Answer from the drawing. Dimensions are ordinates in mm from the lowest x, y and z of the part. A direction names the side the tool comes from. Give positions to 0.01 mm unless a question says otherwise; leave off trailing zeros. Write each loop counter-clockwise with the first axis right and the second up, starting at its lowest first coordinate (ties: lowest second). Pieces come first, ordered by that corner, then holes.
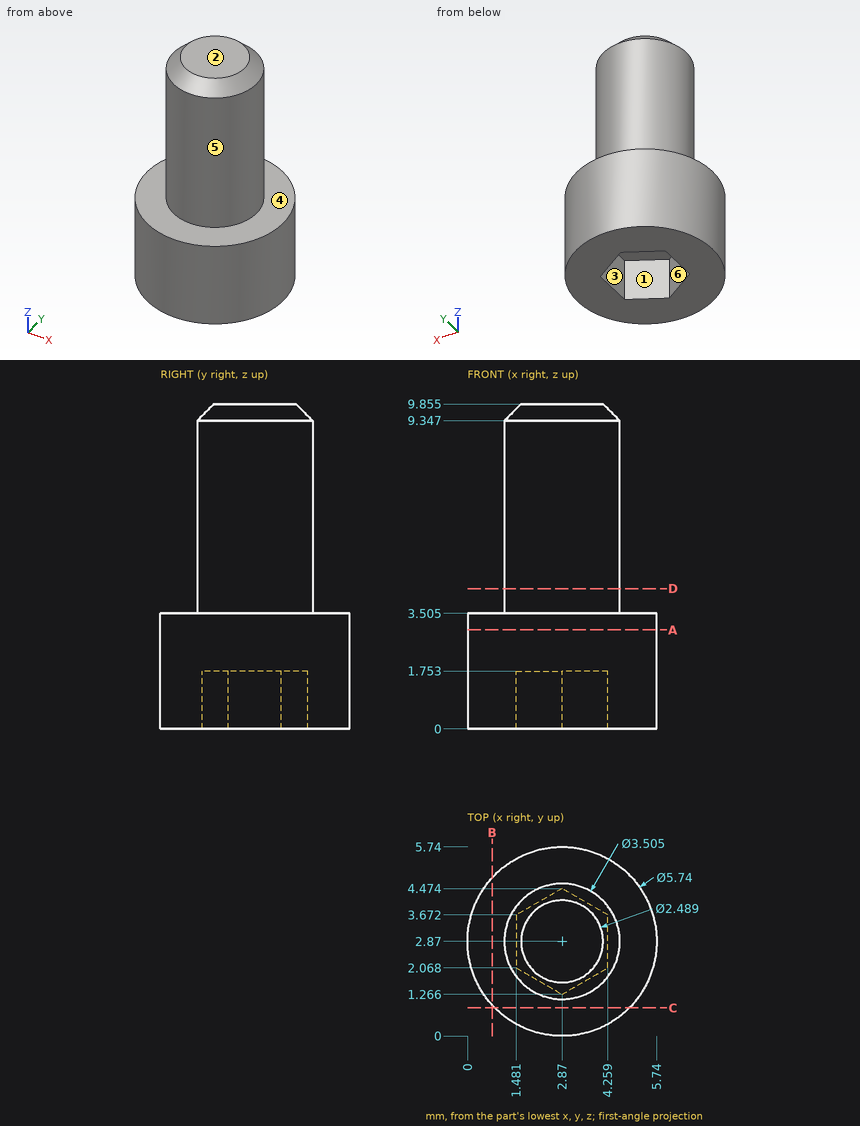
Item 1: A cutting plane is placed at C-C, the plane y = 0.85. Give the vertices of the cut face in (x, z) (1 decimal), plus the area to 3 significant figures.
Conclusion:
outline: (0.8, 0) - (4.9, 0) - (4.9, 3.5) - (0.8, 3.5) - close
area: 14.3 mm2
Item 2: A cutting plane is placed at A-A, the plane z = 3. Give the vertices of the cut face in (x, y), plus the area to 3 significant figures.
Conclusion:
outline: circle Ø5.74 at (2.87, 2.87)
area: 25.9 mm2
Item 3: Determine the mould class of the marked faces 3, 4, 5 and 6 for opening direction Y: pulls with the +Y half, pulls with the -Y half, needs draft (parallel to the pull), parting line crosses it, or undercut.
Conclusion:
face 3: undercut
face 4: needs draft
face 5: parting line crosses it
face 6: undercut
Item 4: A cutting plane is placed at B-B, the plane x = 0.75. Give the vertices of the cut face in (y, z) (1 decimal), plus the area to 3 significant figures.
Conclusion:
outline: (0.9, 0) - (4.8, 0) - (4.8, 3.5) - (0.9, 3.5) - close
area: 13.6 mm2
Item 5: Each of these flat-tipped pins is pushed along its axis until it touches: P1, Ø3, axis at x = 3.5, z = 5.5, coming from the -Y side; P2, Ø1.5, axis at y = 2.5, z = 8.5, coming from the -X side; P3, Ø1, axis at y = 2, z = 5.5, coming from the +X side; P4, Ø1.8, axis at y = 3, z = 0.5, coming from the -X side. Where does it stop, or does it pass through?
Conclusion:
P1: stops at y = 1.12
P2: stops at x = 1.12
P3: stops at x = 4.58
P4: stops at x = 0
Item 6: Which of the six approach directions +Z, -Z, +X, -X, +Y, -Y give full straight-line access (tool end or side, diameter ignored) to the marked faces 1 and 2?
Conclusion:
face 1: -Z
face 2: +Z, +X, -X, +Y, -Y
Item 7: A cutting plane is placed at D-D, the plane z = 4.25. Give the vertices of the cut face in (x, y) (1 decimal).
Conclusion:
outline: circle Ø3.5 at (2.9, 2.9)
Item 8: Consider probe 1 along Z at (x, y) = (3.6, 3.75) (1 decimal); probe 2 along Z at (x, y) = (4.2, 4.95) (1 decimal); probe 3 along X at (y, z) = (2.8, 6.75). Determine where each line is inside the solid, lowest interval first.
Conclusion:
probe 1: z = 1.8 to 9.9
probe 2: z = 0 to 3.5
probe 3: x = 1.12 to 4.62
